Part model, mm, in its own coordinate system. A direction names the side the tool comes from. Give positions to 0.01 mm unless a question says otherwise; leave off trailing zeros. Order: outer loops, then holes, each group sorted by start corner. A loop starts at its lowest first (then second) coordinate and runs counter-clockwise, first axis right, second up. Notation, with made-up numbers: M -16,35 L 9,35 A33 cw 9,72 Z; hole C 40,-24 d6. An arc over 180 degrees is marked long. Return JSON: item names as keys, results as strings.
from build123d import *
from OCP.BRepFilletAPI import BRepFilletAPI_MakeFillet

# Parameters (mm, degrees)
SKETCH_1_R          = 1.7
EXTRUDE_1_DEPTH     = 3
EXTRUDE_2_DEPTH     = 2
FILLET_1_R1         = 3
FILLET_1_R2         = 5
SKETCH_3_R          = 1.2
SKETCH_3_R_2        = 7.5
CUT_EXTRUDE_1_DEPTH = 3


with BuildPart() as part:
    # 草图1 → 凸台-拉伸1 (new body)
    with BuildSketch(Plane.XY):
        with BuildLine():
            Line((0, 17.5), (-20, 17.5))
            Line((-20, 17.5), (-20, -17.5))
            Line((-20, -17.5), (0, -17.5))
            ThreePointArc((0, -17.5), (17.5, 0), (0, 17.5))
        make_face()
        with Locations((-13.5, 0)):
            Circle(SKETCH_1_R, mode=Mode.SUBTRACT)
        with Locations((6.75, 11.691342951)):
            Circle(SKETCH_1_R, mode=Mode.SUBTRACT)
        with Locations((6.75, -11.691342951)):
            Circle(SKETCH_1_R, mode=Mode.SUBTRACT)
    extrude(amount=EXTRUDE_1_DEPTH)

    # 草图2 → 凸台-拉伸2 (add)
    with BuildSketch(Plane.ZY.offset(20)):
        with BuildLine():
            Line((0, -17.5), (50, -17.5))
            ThreePointArc((50, -17.5), (67.5, 0), (50, 17.5))
            Line((50, 17.5), (0, 17.5))
            Line((0, 17.5), (0, -17.5))
        make_face()
    extrude(amount=EXTRUDE_2_DEPTH)

    # 圆角1: one fillet with a radius per group of edges: ONE call of the kernel's fillet builder (fillet() takes one radius for all edges)
    fillet_1_edges_1 = [part.edges().sort_by_distance(p)[0] for p in [
        (-20, 0, 3),
    ]]
    fillet_1_edges_2 = [part.edges().sort_by_distance(p)[0] for p in [
        (-22, 0, 0),
    ]]
    fillet_1 = BRepFilletAPI_MakeFillet(part.part.solid().wrapped)
    for e in fillet_1_edges_1:
        fillet_1.Add(FILLET_1_R1, e.wrapped)
    for e in fillet_1_edges_2:
        fillet_1.Add(FILLET_1_R2, e.wrapped)
    add(Compound.cast(fillet_1.Shape()), mode=Mode.REPLACE)

    # 草图3 → 切除-拉伸1 (cut)
    with BuildSketch(Plane(origin=(-20, 0, 0), x_dir=(0, 0, -1), z_dir=(1, 0, 0))):
        with Locations((-41.583465403, -12)):
            Circle(SKETCH_3_R)
        with Locations((-17.583465403, -12)):
            Circle(SKETCH_3_R)
        with Locations((-17.583465403, 12)):
            Circle(SKETCH_3_R)
        with Locations((-41.583465403, 12)):
            Circle(SKETCH_3_R)
        with Locations((-29.583465403, 0)):
            Circle(SKETCH_3_R_2)
    extrude(amount=-CUT_EXTRUDE_1_DEPTH, mode=Mode.SUBTRACT)


solid = part.part
Q1. Band-saw the part on D-D (x = -19). Give the cut face in (y, z).
Established:
{"outline": "M -17.5,0.42 L 17.5,0.42 L 17.5,3.76 L -17.5,3.76 Z"}
Q2. Band-saw the part on A-A (y = 0). Give the cut face in (x, z), then the cut area to 3 significant figures.
Established:
{"outline": "M -22,5 A5 ccw -17,0 L -15.2,0 L -15.2,3 L -17,3 A3 cw -20,6 L -20,22.08 L -22,22.08 Z; M -22,37.08 L -20,37.08 L -20,67.5 L -22,67.5 Z; M -11.8,0 L 17.5,0 L 17.5,3 L -11.8,3 Z", "area": "204 mm²"}
Q3. Two-plate mould, pull along Z, no slides. Class faces 3 (the cylindrical face through (-20.986, -12.46, 40.475)), 4 (the cylindrical face through (-21, 0, 2)), 5 (the cylindrical face through (17.496, -0.385, 1.479)): +Z half, -Z half, draft (parallel to the pull), parting line (faces both ways), or undercut.
Established:
{"face 3": "undercut", "face 4": "-Z half", "face 5": "draft"}
Q4. Band-saw the part on C-C (z = 28.5). Give the cut face in (x, y).
Established:
{"outline": "M -22,-17.5 L -20,-17.5 L -20,-7.42 L -22,-7.42 Z; M -22,7.42 L -20,7.42 L -20,17.5 L -22,17.5 Z"}
Q5. Pin check, flat tips, straight feed: pin 1 (17 mm diameter, centred on x = -6, y = -4.5, fed in from +Z); pin 2 (17.5 mm diameter, centred on y = 8.5, z = 25, fed in from +X); pin 3 (1.9 mm diameter, centred on y = -12, z = 17.58, fed in from -X). Stop position of each tip, or through.
Established:
{"pin 1": "stops at z = 3", "pin 2": "stops at x = -20", "pin 3": "passes through"}
Q6. Band-saw the part on B-B (x = -13.5). Give the cut face in (y, z).
Established:
{"outline": "M -17.5,0 L -1.7,0 L -1.7,3 L -17.5,3 Z; M 1.7,0 L 17.5,0 L 17.5,3 L 1.7,3 Z"}
Q7. Probe line 1 along X through (y, z) = (-9.5, 36.5); line 2 along Z through (x, y) = (-6, -12.5). List the from-to ranges inside material, lowest first.
Established:
{"line 1": "x = -22 to -20", "line 2": "z = 0 to 3"}
Q8. 3-axis set-ups, long thin cutter, end or side, ignore diameter. For faces 1 (the cylindrical face through (-20.986, 11.54, 40.475)), 2 (the flat face through (0, 0, 3)): which of +Z, -Z, +X, -X, +Y, -Y reach the whole face in a straight line?
Established:
{"face 1": "+X, -X", "face 2": "+Z, +X, +Y, -Y"}
